Part model, mm, in its own coordinate system. A direction names the side the tool comes from. Coordinates: 2 decimals unless noted, no trailing zeros. Loops run counter-clockwise (first coordinate to the right, second up) from the corner with the lowest first, then second, coordinate; pieces in that order, holes last. Notation, with made-up numbers: (83, 44.5) - (118, 44.5) arc R19 cw to (118, 55.5) - close; hole circle Ø3 at (-26.5, -25.5). An arc over 180 degrees is marked (long way). Use a Markdown table: item, result. Add a question column.
1. Wall check: probe 1 along Y at (x, z) = (0, 45.7); probe 2 along Z at (x, y) = (4.25, -1.25); probe 3 along Y at (x, z) = (1, 19.5). Give the ranges that are in metal, low to high. Write a range as [from, to].
2. Band-saw the part on A-A, the plane z = 45. Give the cut face in (x, y), plus the area to 3 significant figures.
3. Pull direction Y, two halves, no side cores. Call faces 4 (the flat face through (4.207, 4.278, 47.686)), 5 (the cylindrical face through (0, 2, 55)), 6 (the flat face through (0, -9, 42.7)), 7 (the flat face through (0, -7.75, 16)): pulls with the +Y half, pulls with the -Y half, needs draft (parallel to the pull), parting line crosses it, or undercut.
4. Band-saw the part on D-D, the plane z = 38. Give the cut face in (x, y).
5. Band-saw the part on B-B, the plane x = 0. Give the cut face in (y, z), plus the area to 3 significant figures.
6. Band-saw the part on C-C, the plane y = -3. Give the cut face in (x, z), plus the area to 3 significant figures.
7. 3-axis set-ups, long thin cutter, end or side, ignore diameter. For faces 1 (the flat face through (0, 7.75, 16)), 2 (the flat face through (-4.207, -4.278, 47.686)), 3 (the cylindrical face through (10.25, 0.12, 15.92)): which of +Z, -Z, +X, -X, +Y, -Y reach the whole face in a straight line?
8. Drop flat-ended pins along their axis: pin 1 (1.6 mm diameter, centred on x = 9.5, y = 0.5, fed in from +Z); pin 2 (1.5 mm diameter, centred on y = 6.5, z = 50, fed in from -X); pin 3 (3 mm diameter, centred on y = 6, z = 33, fed in from -X); pin 4 (4 mm diameter, centred on x = 1, z = 16.5, fed in from -Y). Give the stop position or say it passes through.
from build123d import *

# Parameters (mm, degrees)
BOSS_EXTRU_1_DEPTH      = 32.3
ESQUISSE2_R             = 11
BOSS_EXTRU_2_DEPTH      = 14.4
BOSS_EXTRU_3_DEPTH      = 2
ESQUISSE5_R             = 2
BOSS_EXTRU_4_DEPTH      = 12
ESQUISSE6_R             = 1
ENL_V_MAT_EXTRU_1_DEPTH = 4


with BuildPart() as part:
    # Esquisse1 → Boss.-Extru.1 (new body)
    with BuildSketch(Plane.XY):
        with BuildLine():
            Line((6.708203932, -7.75), (-6.708203932, -7.75))
            ThreePointArc((-6.708203932, -7.75), (-10.25, 0), (-6.708203932, 7.75))
            Line((-6.708203932, 7.75), (6.708203932, 7.75))
            ThreePointArc((6.708203932, 7.75), (10.25, 0), (6.708203932, -7.75))
        make_face()
    extrude(amount=BOSS_EXTRU_1_DEPTH)

    # Esquisse2 → Boss.-Extru.2 (add)
    with BuildSketch(Plane.XY.offset(32.3)):
        Circle(ESQUISSE2_R)
    extrude(amount=BOSS_EXTRU_2_DEPTH)

    # Esquisse4 → Boss.-Extru.3 (add)
    with BuildSketch(Plane.XY.offset(46.7)):
        with BuildLine():
            Line((-1.69313093, -6.792150444), (-6.792150444, -1.69313093))
            ThreePointArc((-6.792150444, -1.69313093), (-4.949747468, 4.949747468), (1.69313093, 6.792150444))
            Line((1.69313093, 6.792150444), (6.792150444, 1.69313093))
            ThreePointArc((6.792150444, 1.69313093), (4.949747468, -4.949747468), (-1.69313093, -6.792150444))
        make_face()
    extrude(amount=BOSS_EXTRU_3_DEPTH)

    # Esquisse5 → Boss.-Extru.4 (add)
    with BuildSketch(Plane.XY.offset(48.7)):
        with Locations(Location((0, 0, 0), (0, 0, 180))):
            Circle(ESQUISSE5_R)
    extrude(amount=BOSS_EXTRU_4_DEPTH)

    # Esquisse6 → Enlèv. mat.-Extru.1 (cut)
    with BuildSketch(Plane.XY.offset(46.7)):
        with Locations((-9, 0)):
            Circle(ESQUISSE6_R)
        with Locations((0, 9)):
            Circle(ESQUISSE6_R)
        with Locations((9, 0)):
            Circle(ESQUISSE6_R)
        with Locations((0, -9)):
            Circle(ESQUISSE6_R)
    extrude(amount=-ENL_V_MAT_EXTRU_1_DEPTH, mode=Mode.SUBTRACT)


solid = part.part
Geometry check:
| question | item | result |
|---|---|---|
| 1 | probe 1 | y = [-11, -10], [-8, 8], [10, 11] |
| 1 | probe 2 | z = [0, 48.7] |
| 1 | probe 3 | y = [-7.75, 7.75] |
| 2 | outline | circle Ø22 at (0, 0); hole circle Ø2 at (-9, 0); hole circle Ø2 at (0, -9); hole circle Ø2 at (0, 9); hole circle Ø2 at (9, 0) |
| 2 | area | 368 mm^2 |
| 3 | face 4 | pulls with the +Y half |
| 3 | face 5 | parting line crosses it |
| 3 | face 6 | undercut |
| 3 | face 7 | pulls with the -Y half |
| 4 | outline | circle Ø22 at (0, 0) |
| 5 | outline | (-11, 32.3) - (-7.75, 32.3) - (-7.75, 0) - (7.75, 0) - (7.75, 32.3) - (11, 32.3) - (11, 46.7) - (10, 46.7) - (10, 42.7) - (8, 42.7) - (8, 46.7) - (7, 46.7) - (7, 48.7) - (2, 48.7) - (2, 60.7) - (-2, 60.7) - (-2, 48.7) - (-7, 48.7) - (-7, 46.7) - (-8, 46.7) - (-8, 42.7) - (-10, 42.7) - (-10, 46.7) - (-11, 46.7) - close |
| 5 | area | 877 mm^2 |
| 6 | outline | (-10.58, 32.3) - (-9.8, 32.3) - (-9.8, 0) - (9.8, 0) - (9.8, 32.3) - (10.58, 32.3) - (10.58, 46.7) - (6.32, 46.7) - (6.32, 48.7) - (-5.49, 48.7) - (-5.49, 46.7) - (-10.58, 46.7) - close |
| 6 | area | 962 mm^2 |
| 7 | face 1 | -Z, +X, -X, +Y |
| 7 | face 2 | +Z, -X, -Y |
| 7 | face 3 | -Z, +X |
| 8 | pin 1 | stops at z = 46.7 |
| 8 | pin 2 | passes through |
| 8 | pin 3 | stops at x = -10.04 |
| 8 | pin 4 | stops at y = -7.75 |
